Can you work these out from the model? Positions are in its coordinate system, mm. Coordinates: 2 decimals unless noted, no trailing zeros. Write each loop counter-clockwise with the first axis right and the second up, starting at its lowest first coordinate (ties: lowest second). Pieces come first, ordered by that corner, then holes. Notation, with made-up numbers: (-3.75, 45.25) - (34.25, 45.25) arc R17 cw to (34.25, 68.25) - close; hole circle Ø6 at (24.5, 65). An arc over 180 degrees is marked (long way). Use one line per item in the form item = value. Start each with the question number.
(1) If we section it at B-B on x = -36.5: Please give me the cut outline in (y, z).
(2) If we section it at C-C on z = 1.8: Give the number of separate pieces and of enclosed holes in the cut face, then the cut area to 3 significant figures.
(3) If I drill on probe 1 along Y at (x, z) = (-37.25, 1.8); probe 2 along Y at (x, z) = (-36.75, 2.85); probe 3 along X at (y, z) = (-30, 2.5) (3 decimals), over which ranges is the centre line in solid material (lowest first)? Write a range as from..to.
(4) If we section it at A-A on y = 20.5: Please give me the cut outline in (x, z), then the cut area to 3 significant figures.
(5) Thinking about a two-plate mould opening in X: for faces 1 (the face through (-53.492, -31.562, 2.028)), 2 (the face through (-45, -45.05, 2)), 3 (the face through (-34.5, 33.81, 2.03)), which applies, pulls with the +X half, pulls with the -X half, needs draft (parallel to the pull), parting line crosses it, or undercut?
```python
from build123d import *

# Parameters (mm, degrees)
SKETCH1_W           = 24
SKETCH1_H           = 80
BOSS_EXTRUDE1_DEPTH = 4
SKETCH2_R           = 4
SKETCH2_R_2         = 1.5
CUT_EXTRUDE1_DEPTH  = 4
FILLET1_R           = 4
SKETCH3_R           = 1.5
CUT_EXTRUDE2_DEPTH  = 4


with BuildPart() as part:
    # Sketch1 → Boss-Extrude1 (new body)
    with BuildSketch(Plane.XY):
        with Locations((-45.296675466, -5.049681021)):
            Rectangle(SKETCH1_W, SKETCH1_H)
    extrude(amount=BOSS_EXTRUDE1_DEPTH)

    # Sketch2 → Cut-Extrude1 (cut)
    with BuildSketch(Plane.XY.offset(4)):
        with Locations((-45.296675466, -33.049681021)):
            Circle(SKETCH2_R)
        with Locations((-37.296675466, -33.049681021)):
            Circle(SKETCH2_R_2)
        with Locations((-45.296675466, -41.049681021)):
            Circle(SKETCH2_R_2)
        with Locations((-53.296675466, -33.049681021)):
            Circle(SKETCH2_R_2)
        with Locations((-45.296675466, -25.049681021)):
            Circle(SKETCH2_R_2)
        with Locations((-45.296675466, 30.950318979)):
            Circle(SKETCH2_R_2)
        with Locations((-37.296675466, 22.950318979)):
            Circle(SKETCH2_R_2)
        with Locations((-45.296675466, 14.950318979)):
            Circle(SKETCH2_R_2)
        with Locations((-53.296675466, 22.950318979)):
            Circle(SKETCH2_R_2)
        with Locations((-45.296675466, 22.950318979)):
            Circle(SKETCH2_R)
    extrude(amount=-CUT_EXTRUDE1_DEPTH, mode=Mode.SUBTRACT)

    # Fillet1
    fillet1_edges = [part.edges().sort_by_distance(p)[0] for p in [
        (-57.296675466, 34.950318979, 2),
        (-57.296675466, -45.049681021, 2),
        (-33.296675466, -45.049681021, 2),
        (-33.296675466, 34.950318979, 2),
    ]]
    fillet(fillet1_edges, radius=FILLET1_R)

    # Sketch3 → Cut-Extrude2 (cut)
    with BuildSketch(Plane.XY.offset(4)):
        with Locations((-45.296675466, -5.049681021)):
            Circle(SKETCH3_R)
    extrude(amount=-CUT_EXTRUDE2_DEPTH, mode=Mode.SUBTRACT)


solid = part.part
```
Reported:
q1.outline = (-44.97, 0) - (-34.32, 0) - (-34.32, 4) - (-44.97, 4) - close; (-31.78, 0) - (21.68, 0) - (21.68, 4) - (-31.78, 4) - close; (24.22, 0) - (34.87, 0) - (34.87, 4) - (24.22, 4) - close
q2.separate_pieces = 1
q2.enclosed_holes = 11
q2.area = 1,740 mm2
q3.probe_1 = -45.05..-34.55, -31.55..21.45, 24.45..34.95
q3.probe_2 = -45.01..-34.45, -31.65..21.55, 24.35..34.91
q3.probe_3 = -57.297..-47.885, -42.708..-33.297
q4.outline = (-57.3, 0) - (-48.46, 0) - (-48.46, 4) - (-57.3, 4) - close; (-42.14, 0) - (-33.3, 0) - (-33.3, 4) - (-42.14, 4) - close
q4.area = 70.7 mm2
q5.face_1 = undercut
q5.face_2 = needs draft
q5.face_3 = pulls with the +X half
